Input: part model. Units: mm. Frame: model coordinates. A direction names the side the tool comes from. Give positions to 0.01 mm unless a question says otherwise; leave off trailing zeros. Loops run counter-clockwise (first coordinate to the right, second up) from the corner with the lowest first, then second, coordinate; pieces in that order, holes last. Notation, with made-up numbers: (57, -24.5) -> (83, -24.5) arc R17 cw to (83, -6.5) -> close; hole circle Ø1 at (30.5, -8.75). An arc over 180 degrees is marked (long way). Answer in a Markdown table with one row per item. Add a question column.
Autodesk Inventor part; units mm, degrees
ref_plane "YZ Plane" through (0, 0, 0) normal (1, 0, 0) x (0, 1, 0)
ref_plane "XZ Plane" through (0, 0, 0) normal (0, 1, 0) x (-1, 0, 0)
ref_plane "XY Plane" through (0, 0, 0) normal (0, 0, 1) x (1, 0, 0)
sketch "Sketch1" plane through (0, 0, 0) normal (0, 0, 1) x (1, 0, 0)
  circle A0 centre (0, 0) radius 7.5
  line L0 (2.5, -2.5) -> (-2.5, -2.5)
  line L1 (-2.5, -2.5) -> (-2.5, 2.5)
  line L2 (-2.5, 2.5) -> (2.5, 2.5)
  line L3 (2.5, 2.5) -> (2.5, -2.5)
  line L4 (2.5, -2.5) -> (-2.5, 2.5) construction
  line L5 (-2.5, -2.5) -> (2.5, 2.5) construction
  dimension "d0" = 15
  dimension "d1" = 5
  dimension "d2" = 5
extrude "Extrusion1" add sketch "Sketch1" along normal blind 10
properties part number "ArmCylinder"
1) Reachability of faces 5 (the face through (0, -2.5, 5)), 6 (the face through (0, -3, 10)) from +Z, -Z, +X, -X, +Y, -Y: full face, straight path, thin tool, end or side. Return the list, or none.
2) Pull-direction query (Y, two-part tool) for faces 1 (the face through (2.5, 0, 5)), 2 (the face through (0, -3, 0)), 3 (the face through (0, 2.5, 5)), 4 (the face through (-7.493, -0.33, 4.93)); classes: +Y half, -Y half, draft (parallel to the pull), parting line (faces both ways), or undercut.
3) Material intervals for line 1 along Y through (x, z) = (-1, 4.75); line 2 along Y through (x, z) = (1.5, 6.5); line 3 along X through (y, z) = (-0.5, 3.5), sorted ascending.
4) Section C-C on z = 4.75. Output: boundary loops of the cut face in (x, y).
5) Section D-D on y = 3.5. Output: boundary loops of the cut face in (x, z).
6) Section A-A on y = 0. Output: boundary loops of the cut face in (x, z).
7) Pin query (flat end, axial travel): pin 1 (2 mm diameter, centred on y = 2.5, z = 5.5, fed in from -X); pin 2 (4 mm diameter, centred on x = 5.5, z = 3, fed in from +Y); pin 3 (2.5 mm diameter, centred on y = 0.5, z = 7, fed in from +X); pin 4 (1.5 mm diameter, centred on x = 2, z = 1.5, fed in from -Y). Return the tip coordinate at first contact, or that it passes through.
Working result:
| question | item | result |
|---|---|---|
| 1 | face 5 | +Z, -Z |
| 1 | face 6 | +Z, +X, -X, +Y, -Y |
| 2 | face 1 | undercut |
| 2 | face 2 | draft |
| 2 | face 3 | undercut |
| 2 | face 4 | parting line |
| 3 | line 1 | y = -7.43 to -2.5, 2.5 to 7.43 |
| 3 | line 2 | y = -7.35 to -2.5, 2.5 to 7.35 |
| 3 | line 3 | x = -7.48 to -2.5, 2.5 to 7.48 |
| 4 | outline | circle Ø15 at (0, 0); hole (-2.5, -2.5) -> (2.5, -2.5) -> (2.5, 2.5) -> (-2.5, 2.5) -> close |
| 5 | outline | (-6.63, 0) -> (6.63, 0) -> (6.63, 10) -> (-6.63, 10) -> close |
| 6 | outline | (-7.5, 0) -> (-2.5, 0) -> (-2.5, 10) -> (-7.5, 10) -> close; (2.5, 0) -> (7.5, 0) -> (7.5, 10) -> (2.5, 10) -> close |
| 7 | pin 1 | stops at x = -7.35 |
| 7 | pin 2 | stops at y = 6.63 |
| 7 | pin 3 | stops at x = 7.5 |
| 7 | pin 4 | stops at y = -7.4 |
